Here's the drawing with two shaded views (mm, measured from the low corner). I have some questions. Round coordinates to 2 decimals unless told otherwise and drop trailing zeros. Loops run counter-clockwise (first coordinate to the right, second up) from the corner with the lowest first, then second, coordinate; pieces in that order, holes last. Notation, with made-up numbers: M 83,-3 L 126,-3 A20 cw 126,27 Z; hole C -6.75,36 d9. An arc over 180 degrees is marked long. One line per item, written item: value. Start each with the question number.
Q1. Please list where these lines run through material, in increasing order: line 1 along Y through (x, z) = (22, 2); line 2 along X through (y, z) = (14, 20.5) (1 decimal); line 3 along Z through (x, y) = (24, 4.75).
Q2. Imagine slicing it at A-A (x = 17). Please give me the cut outline in (y, z).
Q3. Imagine slicing it at D-D (x = 11.5). Please give me the cut outline in (y, z) (1 decimal).
Q4. Imagine slicing it at B-B (y = 3.75). Please give me the cut outline in (x, z), then the cut area to 3 significant figures.
Q5. Imagine slicing it at C-C (y = 1.5). Please give me the cut outline in (x, z), then the cut area to 3 significant figures.
Q6. I'm going to push flat-ended pins straight in: pin 1 Ø3.5 at (x, z) = (19, 27.5) entering from +Y; pin 2 Ø8 at (x, y) = (6.5, 10) entering from -Z; pin 3 Ø9.5 at (x, y) = (23.5, 12.5) entering from +Z; pin 4 Ø10 at (y, z) = (13, 14) entering from -X. Where does each tip first touch, or does it pass through?
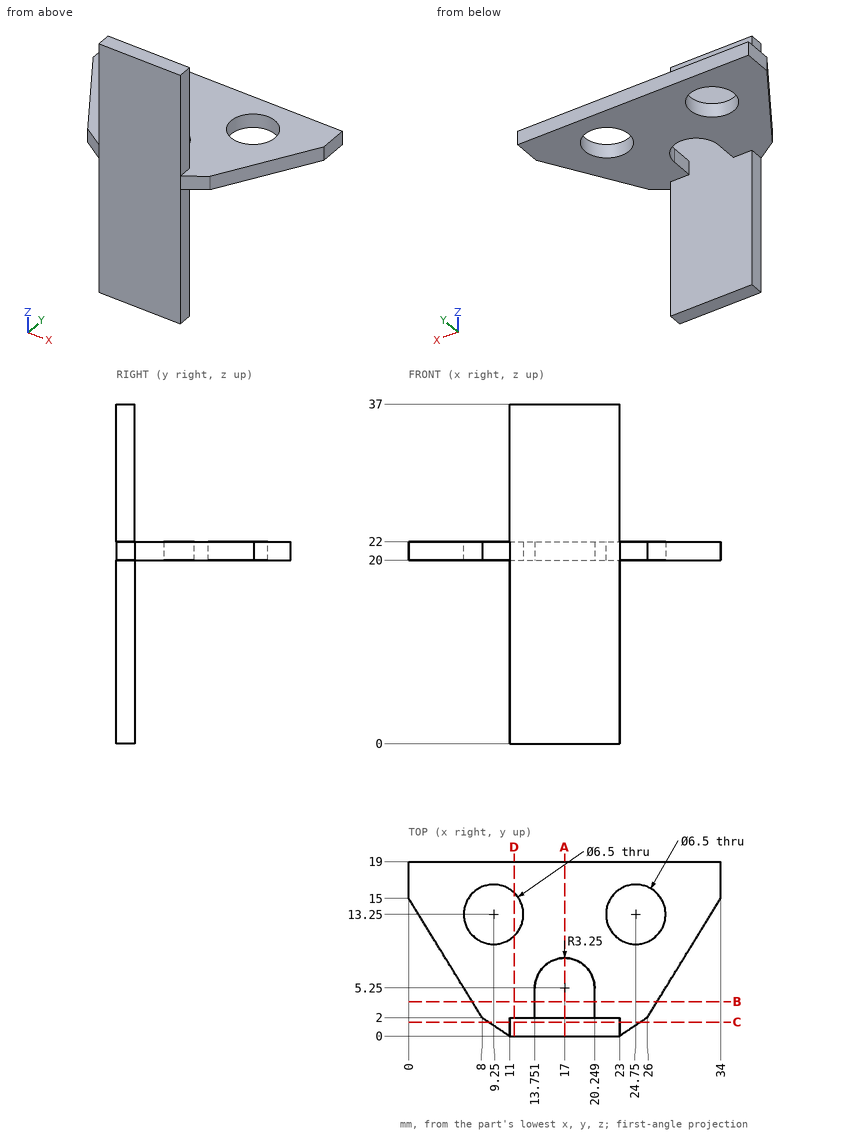
Report:
1. line 1: y = 0 to 2
1. line 2: x = 0.6 to 6.1, 12.4 to 21.6, 27.9 to 33.4
1. line 3: z = 20 to 22
2. outline: M 0,0 L 2,0 L 2,37 L 0,37 Z; M 8.5,20 L 19,20 L 19,22 L 8.5,22 Z
3. outline: M 0,0 L 2,0 L 2,20 L 10.9,20 L 10.9,22 L 2,22 L 2,37 L 0,37 Z; M 15.6,20 L 19,20 L 19,22 L 15.6,22 Z
4. outline: M 6.92,20 L 13.75,20 L 13.75,22 L 6.92,22 Z; M 20.25,20 L 27.08,20 L 27.08,22 L 20.25,22 Z
4. area: 27.3 mm²
5. outline: M 8.75,20 L 11,20 L 11,0 L 23,0 L 23,20 L 25.25,20 L 25.25,22 L 23,22 L 23,37 L 11,37 L 11,22 L 8.75,22 Z
5. area: 453 mm²
6. pin 1: stops at y = 2
6. pin 2: stops at z = 20
6. pin 3: stops at z = 22
6. pin 4: passes through
